Could you check a few things on this model? Use its own coordinates, in mm. A direction names the side the tool comes from. Give positions to 0.01 mm unless a question says otherwise; leave off trailing zeros. Order: outer loops, then holes, each group sorted by start corner. A loop starts at its lowest first (then second) coordinate and runs counter-clockwise, first axis right, second up. Notation, with made-up numbers: (14.25, -36.75) - (25.25, -36.75) arc R32 cw to (25.25, -3.75) - close; hole circle Ø2 at (40.5, -24). An arc over 180 degrees is marked (long way). Put each result on its own line as item: value.
Autodesk Inventor part; units mm, degrees
ref_plane "YZ Plane" through (0, 0, 0) normal (1, 0, 0) x (0, 1, 0)
ref_plane "XZ Plane" through (0, 0, 0) normal (0, 1, 0) x (-1, 0, 0)
ref_plane "XY Plane" through (0, 0, 0) normal (0, 0, 1) x (1, 0, 0)
sketch "Sketch1" plane through (0, 0, 0) normal (0, 0, 1) x (1, 0, 0)
  line L0 (-32.75, 32.75) -> (32.75, 32.75)
  line L1 (32.75, 32.75) -> (32.75, -32.75)
  line L2 (32.75, -32.75) -> (-32.75, -32.75)
  line L3 (-32.75, -32.75) -> (-32.75, 32.75)
  line L4 (0, 32.75) -> (0, -32.75) construction
  line L5 (-32.75, 0) -> (32.75, 0) construction
  point P0 (0, 0)
  dimension "d0" = 65.5
  dimension "d1" = 65.5
extrude "Extrusion1" add sketch "Sketch1" along normal blind 3
sketch "Sketch2" plane through (0, 0, 3) normal (0, 0, 1) x (1, 0, 0)
  line L0 (32.75, 32.75) -> (-32.75, 32.75)
  line L1 (-32.75, 32.75) -> (-32.75, -32.75)
  line L2 (-32.75, -32.75) -> (32.75, -32.75)
  line L3 (32.75, -32.75) -> (32.75, 32.75)
  circle A0 centre (0, 0) radius 2.5
  circle A1 centre (0, 10) radius 2.5
  line L4 (0, 0) -> (0, 20.5611) construction
  circle A2 centre (-10, 0) radius 2.5
  circle A3 centre (0, -10) radius 2.5
  circle A4 centre (10, 0) radius 2.5
  circle A5 centre (-19.85, 0) radius 2.5
  circle A6 centre (-19.85, -10) radius 2.5
  circle A7 centre (-19.85, -20) radius 2.5
  circle A8 centre (-19.85, 10) radius 2.5
  circle A9 centre (-19.85, 0) radius 2.5
  circle A10 centre (-19.85, -10) radius 2.5
  circle A11 centre (-19.85, 20) radius 2.5
  circle A12 centre (-19.85, 10) radius 2.5
  circle A13 centre (-19.85, 0) radius 2.5
  line L5 (19.85, 32.75) -> (19.85, -32.75) construction
  circle A14 centre (19.85, 10) radius 2.5
  circle A15 centre (19.85, -10) radius 2.5
  line L6 (0, 0) -> (-32.75, 0) construction
  circle A16 centre (19.85, 0) radius 3.6
  circle A17 centre (19.85, 20) radius 3.6
  circle A18 centre (19.85, -20) radius 3.6
  circle A19 centre (19.85, 0) radius 3.6
  dimension "d4" = 5
  dimension "d5" = 5
  dimension "d6" = 10
  dimension "d9" = 360
  dimension "d11" = 5
  dimension "d12" = 12.9
  dimension "d15" = 10
  dimension "d18" = 10
  dimension "d21" = 5
  dimension "d22" = 5
  dimension "d23" = 12.9
  dimension "d24" = 10
  dimension "d25" = 7.2
  dimension "d28" = 20
  dimension "d31" = 20
extrude "Extrusion2" cut sketch "Sketch2" against normal up to next contours A0 | A1 | A2 | A3 | A4 | A5 | A6 | A7 | A8 | A11 | A14 | A15 | A16 | A17 | A18
sketch "Sketch3" plane through (0, 0, 3) normal (0, 0, 1) x (1, 0, 0)
  circle A0 centre (-19.85, -20) radius 2.5
  circle A1 centre (0, 0) radius 2.5
  line L0 (32.75, 32.75) -> (-32.75, 32.75)
  line L1 (-32.75, -32.75) -> (32.75, -32.75)
  line L2 (-10.32, -20) -> (10.32, -20) construction
  line L3 (-10.32, -22.5) -> (10.32, -22.5)
  line L4 (10.32, -17.5) -> (-10.32, -17.5)
  arc A2 (-10.32, -17.5) -> (-10.32, -22.5) centre (-10.32, -20) ccw
  arc A3 (10.32, -22.5) -> (10.32, -17.5) centre (10.32, -20) ccw
  line L5 (0, 0) -> (0, -39.6664) construction
  line L6 (0, 0) -> (-44.4767, 0) construction
  line L7 (-10.32, 20) -> (10.32, 20) construction
  line L8 (-10.32, 22.5) -> (10.32, 22.5)
  line L9 (10.32, 17.5) -> (-10.32, 17.5)
  arc A4 (-10.32, 22.5) -> (-10.32, 17.5) centre (-10.32, 20) ccw
  arc A5 (10.32, 17.5) -> (10.32, 22.5) centre (10.32, 20) ccw
  line L10 (-3.25, -27.7) -> (3.25, -27.7) construction
  line L11 (-3.25, -29.2) -> (3.25, -29.2)
  line L12 (3.25, -26.2) -> (-3.25, -26.2)
  arc A6 (-3.25, -26.2) -> (-3.25, -29.2) centre (-3.25, -27.7) ccw
  arc A7 (3.25, -29.2) -> (3.25, -26.2) centre (3.25, -27.7) ccw
  line L13 (16.9, -27.7) -> (23.4, -27.7) construction
  line L14 (16.9, -29.2) -> (23.4, -29.2)
  line L15 (23.4, -26.2) -> (16.9, -26.2)
  arc A8 (16.9, -26.2) -> (16.9, -29.2) centre (16.9, -27.7) ccw
  arc A9 (23.4, -29.2) -> (23.4, -26.2) centre (23.4, -27.7) ccw
  line L16 (-23.4, -27.7) -> (-16.9, -27.7) construction
  line L17 (-23.4, -29.2) -> (-16.9, -29.2)
  line L18 (-16.9, -26.2) -> (-23.4, -26.2)
  arc A10 (-23.4, -26.2) -> (-23.4, -29.2) centre (-23.4, -27.7) ccw
  arc A11 (-16.9, -29.2) -> (-16.9, -26.2) centre (-16.9, -27.7) ccw
  line L19 (-3.25, -27.7) -> (3.25, -27.7) construction
  line L20 (-3.25, -29.2) -> (3.25, -29.2)
  line L21 (3.25, -26.2) -> (-3.25, -26.2)
  arc A12 (-3.25, -26.2) -> (-3.25, -29.2) centre (-3.25, -27.7) ccw
  arc A13 (3.25, -29.2) -> (3.25, -26.2) centre (3.25, -27.7) ccw
  line L22 (-3.25, 27.7) -> (3.25, 27.7) construction
  line L23 (-3.25, 29.2) -> (3.25, 29.2)
  line L24 (3.25, 26.2) -> (-3.25, 26.2)
  arc A14 (-3.25, 29.2) -> (-3.25, 26.2) centre (-3.25, 27.7) ccw
  arc A15 (3.25, 26.2) -> (3.25, 29.2) centre (3.25, 27.7) ccw
  arc A16 (16.9, 29.2) -> (16.9, 26.2) centre (16.9, 27.7) ccw
  line L25 (23.4, 26.2) -> (16.9, 26.2)
  line L26 (16.9, 27.7) -> (23.4, 27.7) construction
  line L27 (16.9, 29.2) -> (23.4, 29.2)
  arc A17 (23.4, 26.2) -> (23.4, 29.2) centre (23.4, 27.7) ccw
  arc A18 (-23.4, 29.2) -> (-23.4, 26.2) centre (-23.4, 27.7) ccw
  line L28 (-16.9, 26.2) -> (-23.4, 26.2)
  line L29 (-23.4, 27.7) -> (-16.9, 27.7) construction
  line L30 (-23.4, 29.2) -> (-16.9, 29.2)
  arc A19 (-16.9, 26.2) -> (-16.9, 29.2) centre (-16.9, 27.7) ccw
  arc A20 (-3.25, 29.2) -> (-3.25, 26.2) centre (-3.25, 27.7) ccw
  line L31 (3.25, 26.2) -> (-3.25, 26.2)
  line L32 (-3.25, 27.7) -> (3.25, 27.7) construction
  line L33 (-3.25, 29.2) -> (3.25, 29.2)
  arc A21 (3.25, 26.2) -> (3.25, 29.2) centre (3.25, 27.7) ccw
  point P0 (0, -20)
  point P1 (0, 20)
  point P2 (0, -27.7)
  point P3 (20.15, -27.7)
  point P4 (-20.15, -27.7)
  point P5 (0, -27.7)
  point P6 (0, 27.7)
  point P7 (20.15, 27.7)
  point P8 (-20.15, 27.7)
  point P9 (0, 27.7)
  dimension "d36" = 5
  dimension "d37" = 20.64
  dimension "d38" = 3
  dimension "d39" = 60.45
  dimension "d40" = 6.5
  dimension "d43" = 20.15
  dimension "d46" = 20.15
extrude "Extrusion3" cut sketch "Sketch3" against normal up to next contours A2 L4 A3 L3 | L8 A5 L9 A4 | A6 L12 A7 L11 | A8 L15 A9 L14 | A10 L18 A11 L17 | L23 A15 L24 A14 | L27 A17 L25 A16 | L30 A19 L28 A18
fillet "Fillet1" radius 3.38 4 edges at (32.75, -32.75, 1.5) (32.75, 32.75, 1.5) (-32.75, -32.75, 1.5) (-32.75, 32.75, 1.5)
properties part number "20mm gantry plate"
1) I'm going to push a flat-ended pin straight in: pin 1 (3 mm diameter, centred on x = 10, y = 0, fed in from -Z). Where does the tip first touch, or does it pass through?
Filled in:
pin 1: passes through
2) If I drill on line 1 (Y direction, x = 5, z = 1.2); line 2 (Y direction, x = 10, z = 1.15); line 3 (X direction, y = -1.5, z = 0.7), over which ranges is the centre line in solid material (lowest first)? Write a range as [from, to].
Filled in:
line 1: y = [-32.75, -22.5], [-17.5, 17.5], [22.5, 32.75]
line 2: y = [-32.75, -22.5], [-17.5, -2.5], [2.5, 17.5], [22.5, 32.75]
line 3: x = [-32.75, -21.85], [-17.85, -12], [-8, -2], [2, 8], [12, 16.58], [23.12, 32.75]
3) Suppose I cut it at A-A, the plane y = -27.7. List the corners of the cut face in (x, z) for me, and give its area (3 significant figures).
Filled in:
outline: (-32.75, 0) - (-24.9, 0) - (-24.9, 3) - (-32.75, 3) - close; (-15.4, 0) - (-4.75, 0) - (-4.75, 3) - (-15.4, 3) - close; (4.75, 0) - (15.4, 0) - (15.4, 3) - (4.75, 3) - close; (24.9, 0) - (32.75, 0) - (32.75, 3) - (24.9, 3) - close
area: 111 mm^2
4) Suppose I cut it at C-C, the plane y = 10. List the corners of the cut face in (x, z) for me.
Filled in:
outline: (-32.75, 0) - (-22.35, 0) - (-22.35, 3) - (-32.75, 3) - close; (-17.35, 0) - (-2.5, 0) - (-2.5, 3) - (-17.35, 3) - close; (2.5, 0) - (17.35, 0) - (17.35, 3) - (2.5, 3) - close; (22.35, 0) - (32.75, 0) - (32.75, 3) - (22.35, 3) - close
5) We'd pull the mould along Y, two halves only. Please class faces 1 (the cylindrical face through (31.73, -31.79, 1.52)), 2 (the cylindrical face through (-31.73, 31.79, 1.52)), 3 (the cylindrical face through (7.5, 0.1, 1.5)): pulls with the +Y half, pulls with the -Y half, needs draft (parallel to the pull), parting line crosses it, or undercut.
Filled in:
face 1: pulls with the -Y half
face 2: pulls with the +Y half
face 3: undercut
6) Suppose I cut it at B-B, the plane x = 0. State how many separate pieces and enclosed holes the cut face has, and give its area (4 significant figures).
Filled in:
separate pieces: 8
enclosed holes: 0
area: 103.5 mm^2
7) Which directions (+Z, -Z, +X, -X, +Y, -Y) give clear straight access to the entire face, cutting with the end or side of a thin tool? Please do faces 4 (the cylindrical face through (15.4, 27.7, 1.5)), 5 (the flat face through (32.75, 0, 1)).
Filled in:
face 4: +Z, -Z
face 5: +Z, -Z, +X, +Y, -Y
